from build123d import *

# Parameters (mm, degrees)
SKETCH1_W           = 90
SKETCH1_H           = 38.1
BOSS_EXTRUDE1_DEPTH = 3.175
SKETCH2_R           = 2.35
SKETCH2_W           = 41
SKETCH2_H           = 21
CUT_EXTRUDE1_DEPTH  = 49.969205885
FILLET1_R           = 2
CUT_EXTRUDE2_DEPTH  = 49.969205885


with BuildPart() as part:
    # Sketch1 → Boss-Extrude1 (new body)
    with BuildSketch(Plane(origin=(0, 0, 0), x_dir=(1, 0, 0), z_dir=(0, 1, 0))):
        Rectangle(SKETCH1_W, SKETCH1_H)
    extrude(amount=BOSS_EXTRUDE1_DEPTH)

    # Sketch2 → Cut-Extrude1 (cut, through all)
    with BuildSketch(Plane(origin=(0, 3.175, 0), x_dir=(1, 0, 0), z_dir=(0, 1, 0))):
        with Locations(Location((-25.25, 5, 0), (0, 0, 270))):
            Circle(SKETCH2_R)
        with Locations(Location((-25.25, -5.503329438, 0), (0, 0, 270))):
            Circle(SKETCH2_R)
        with Locations(Location((25.25, 5, 0), (0, 0, 90))):
            Circle(SKETCH2_R)
        with Locations(Location((25.25, -5.503329438, 0), (0, 0, 90))):
            Circle(SKETCH2_R)
        Rectangle(SKETCH2_W, SKETCH2_H)
    extrude(amount=-CUT_EXTRUDE1_DEPTH, mode=Mode.SUBTRACT)

    # Fillet1
    fillet1_edges = [part.edges().sort_by_distance(p)[0] for p in [
        (-20.5, 1.5875, 10.5),
        (-20.5, 1.5875, -10.5),
        (20.5, 1.5875, -10.5),
        (20.5, 1.5875, 10.5),
        (-45, 1.5875, -19.05),
        (45, 1.5875, -19.05),
        (45, 1.5875, 19.05),
        (-45, 1.5875, 19.05),
    ]]
    fillet(fillet1_edges, radius=FILLET1_R)

    # Sketch3 → Cut-Extrude2 (cut, through all)
    with BuildSketch(Plane(origin=(0, 3.175, 0), x_dir=(1, 0, 0), z_dir=(0, 1, 0))):
        with BuildLine():
            Line((-36.475, 10.670041553), (-36.475, -11.329958447))
            ThreePointArc((-36.475, -11.329958447), (-38, -12.854958447), (-39.525, -11.329958447))
            Line((-39.525, -11.329958447), (-39.525, 10.670041553))
            ThreePointArc((-39.525, 10.670041553), (-38, 12.195041553), (-36.475, 10.670041553))
        make_face()
        with BuildLine():
            Line((36.475, 10.670041553), (36.475, -11.329958447))
            ThreePointArc((36.475, -11.329958447), (38, -12.854958447), (39.525, -11.329958447))
            Line((39.525, -11.329958447), (39.525, 10.670041553))
            ThreePointArc((39.525, 10.670041553), (38, 12.195041553), (36.475, 10.670041553))
        make_face()
    extrude(amount=-CUT_EXTRUDE2_DEPTH, mode=Mode.SUBTRACT)


solid = part.part
Source: CAD feature listing. Evaluate the final solid. Frame: model axes, mm. A direction names the side the tool comes from. Give positions to 0.01 mm unless a question says otherwise; leave off trailing zeros. Order: outer loops, then holes, each group sorted by start corner. A loop starts at its lowest first (then second) coordinate and runs counter-clockwise, first axis right, second up. Notation, with made-up numbers: (88.25, 70) -> (107.25, 70) arc R20 ccw to (107.25, 104) -> close; hole circle Ø7 at (62.25, -12.5). An arc over 180 degrees is marked (long way). Use a Markdown table: item, result.
1) Section query B-B, the plane z = -5. Return the cut outline in (x, y) (3 decimals), then the cut area to 3 significant figures.
Answer list:
| item | result |
|---|---|
| outline | (-45, 0) -> (-39.525, 0) -> (-39.525, 3.175) -> (-45, 3.175) -> close; (-36.475, 0) -> (-27.6, 0) -> (-27.6, 3.175) -> (-36.475, 3.175) -> close; (-22.9, 0) -> (-20.5, 0) -> (-20.5, 3.175) -> (-22.9, 3.175) -> close; (20.5, 0) -> (22.9, 0) -> (22.9, 3.175) -> (20.5, 3.175) -> close; (27.6, 0) -> (36.475, 0) -> (36.475, 3.175) -> (27.6, 3.175) -> close; (39.525, 0) -> (45, 0) -> (45, 3.175) -> (39.525, 3.175) -> close |
| area | 106 mm² |
2) Section query C-C, the plane x = -25.25. Return the cut outline in (y, z) (3 decimals).
Answer list:
| item | result |
|---|---|
| outline | (0, -19.05) -> (3.175, -19.05) -> (3.175, -7.35) -> (0, -7.35) -> close; (0, -2.65) -> (3.175, -2.65) -> (3.175, 3.153) -> (0, 3.153) -> close; (0, 7.853) -> (3.175, 7.853) -> (3.175, 19.05) -> (0, 19.05) -> close |
3) Mould query, pull axis Z, two halves, no side actions, for faces 3 (the cylindrical face through (-44.43, 1.61, -18.45)), 4 (the flat face through (0, 2, -10.5)), 5 (the flat face through (-11, 3.175, -13)), 6 (the flat face through (-1, 2, 19.05)). Classes: +Z half, -Z half, draft (parallel to the pull), parting line (faces both ways), or undercut.
Answer list:
| item | result |
|---|---|
| face 3 | -Z half |
| face 4 | undercut |
| face 5 | draft |
| face 6 | +Z half |
4) Section query A-A, the plane x = -13. Return the cut outline in (y, z) (3 decimals).
Answer list:
| item | result |
|---|---|
| outline | (0, -19.05) -> (3.175, -19.05) -> (3.175, -10.5) -> (0, -10.5) -> close; (0, 10.5) -> (3.175, 10.5) -> (3.175, 19.05) -> (0, 19.05) -> close |
5) Section query D-D, the plane y = 0.8. Return the cut outline in (x, z) (3 decimals), then the cut area to 3 significant figures.
Answer list:
| item | result |
|---|---|
| outline | (-45, -17.05) arc R2 ccw to (-43, -19.05) -> (43, -19.05) arc R2 ccw to (45, -17.05) -> (45, 17.05) arc R2 ccw to (43, 19.05) -> (-43, 19.05) arc R2 ccw to (-45, 17.05) -> close; hole (-39.525, -10.67) arc R1.525 ccw to (-36.475, -10.67) -> (-36.475, 11.33) arc R1.525 ccw to (-39.525, 11.33) -> close; hole circle Ø4.7 at (-25.25, -5); hole circle Ø4.7 at (-25.25, 5.503); hole (-20.5, -8.5) arc R2 ccw to (-18.5, -10.5) -> (18.5, -10.5) arc R2 ccw to (20.5, -8.5) -> (20.5, 8.5) arc R2 ccw to (18.5, 10.5) -> (-18.5, 10.5) arc R2 ccw to (-20.5, 8.5) -> close; hole circle Ø4.7 at (25.25, -5); hole circle Ø4.7 at (25.25, 5.503); hole (36.475, -10.67) arc R1.525 ccw to (39.525, -10.67) -> (39.525, 11.33) arc R1.525 ccw to (36.475, 11.33) -> close |
| area | 2,350 mm² |
6) Ray query, line 1 along X through (y, z) = (0.2, 0) (3 decimals); line 2 along X through (y, z) = (1.5, -5) (3 decimals); line 3 along Z through (x, y) = (25.25, 0.85). Return the intervals inside material, ascending. Write a range as [from, to].
Answer list:
| item | result |
|---|---|
| line 1 | [-45, -39.525], [-36.475, -20.5], [20.5, 36.475], [39.525, 45] |
| line 2 | [-45, -39.525], [-36.475, -27.6], [-22.9, -20.5], [20.5, 22.9], [27.6, 36.475], [39.525, 45] |
| line 3 | [-19.05, -7.35], [-2.65, 3.15], [7.85, 19.05] |
7) Contact query for a flat-ended pin moving along its axis: P1, Ø6, axis at x = -25.25, z = -5, coming from the -Y side. Output: stop coordinate, or through.
Answer list:
| item | result |
|---|---|
| P1 | y = 0 |
8) Reachability of faces 1 (the cylindrical face through (44.4, 1.61, -18.48)), 2 (the flat face through (39.525, 2, 0)) from +Z, -Z, +X, -X, +Y, -Y: full face, straight path, thin tool, end or side. Return the list, or none.
Answer list:
| item | result |
|---|---|
| face 1 | -Z, +X, +Y, -Y |
| face 2 | +Y, -Y |
